```python
from build123d import *

# Parameters (mm, degrees)
SKETCH2_W             = 450.0499
SKETCH2_H             = 50.8
BOSS_EXTRUDE1_DEPTH   = 3.175
F_8_32_TAPPED_HOLE1_D = 3.4544
SKETCH5_W             = 6.096
SKETCH5_H             = 12.7
CUT_EXTRUDE1_DEPTH    = 227.542955358


with BuildPart() as part:
    # Sketch2 → Boss-Extrude1 (new, symmetric)
    with BuildSketch(Plane.XY):
        Rectangle(SKETCH2_W, SKETCH2_H)
    extrude(amount=BOSS_EXTRUDE1_DEPTH, both=True)

    # #8-32 Tapped Hole1 (through all)
    with Locations(Plane.XY.offset(3.175)):
        with Locations((-212.32495, 12.7), (-212.32495, -12.7), (212.32495, 12.7), (212.32495, -12.7), (-186.92495, 12.7), (-186.92495, -12.7), (186.92495, 12.7), (186.92495, -12.7)):
            Hole(F_8_32_TAPPED_HOLE1_D / 2)

    # Sketch5 → Cut-Extrude1 (cut, through all)
    with BuildSketch(Plane.XY.offset(3.175)):
        with Locations((-104.648, 12.7)):
            Rectangle(SKETCH5_W, SKETCH5_H)
        with Locations((-104.648, -12.7)):
            Rectangle(SKETCH5_W, SKETCH5_H)
        with Locations((104.648, 12.7)):
            Rectangle(SKETCH5_W, SKETCH5_H)
        with Locations((104.648, -12.7)):
            Rectangle(SKETCH5_W, SKETCH5_H)
    extrude(amount=-CUT_EXTRUDE1_DEPTH, mode=Mode.SUBTRACT)


solid = part.part
```
Input: part model. Units: mm. Frame: model coordinates. Coordinates: 2 decimals unless noted, no trailing zeros. Answer in a Markdown table with one row per item.
(1) Material intervals for L1, parallel to X at y = 19, z = -2.75, sorted ascending. Write a range as from..to.
Model answer:
| item | result |
|---|---|
| L1 | x = -225.02..-107.7, -101.6..101.6, 107.7..225.02 |
(2) Cut plane A-A on z = -2. Count the separate pieces of the cut face and the enclosed holes in it, plus the area to 3 significant figures.
Model answer:
| item | result |
|---|---|
| separate pieces | 1 |
| enclosed holes | 12 |
| area | 22,500 mm² |
(3) Pin query (flat end, axial travel): P1, Ø3, axis at x = 186.92, y = 12.7, coming from the +Z side. Return the tip coordinate at first contact, or that it passes through.
Model answer:
| item | result |
|---|---|
| P1 | passes through |
